Geometry check sheet. Reference: the model listing, model coordinates, mm. A direction names the side the tool comes from. Round coordinates to 2 decimals unless told otherwise and drop trailing zeros. Loops run counter-clockwise (first coordinate to the right, second up) from the corner with the lowest first, then second, coordinate; pieces in that order, holes last. Notation, with made-up numbers: (58.25, 81.5) -> (67.25, 81.5) arc R22 cw to (67.25, 94.5) -> close; hole circle Ø6 at (21, 14.25). An arc over 180 degrees is marked (long way). Use one line per item in the form item = value.
from build123d import *

# Parameters (mm, degrees)
F1_DEPTH = 25.4
F3_DEPTH = 3.176


with BuildPart() as f1:
    # F0 (on Front) → F1 (new body)
    with BuildSketch(Plane.XZ):
        with BuildLine():
            ThreePointArc((3.175, 3.175), (0.929936, 2.245064), (0, 0))
            Line((0, 0), (76.2, 0))
            Line((76.2, 0), (76.2, 76.2))
            ThreePointArc((76.2, 76.2), (73.954936, 75.270064), (73.025, 73.025))
            Line((73.025, 73.025), (73.025, 6.35))
            ThreePointArc((73.025, 6.35), (72.095064, 4.104936), (69.85, 3.175))
            Line((69.85, 3.175), (3.175, 3.175))
        make_face()
    extrude(amount=F1_DEPTH)

    # F2 (on face) → F3 (cut, through all)
    with BuildSketch(Plane.XY.offset(3.175)):
        with BuildLine():
            Line((55.5625, -9.525), (17.4625, -9.525))
            ThreePointArc((17.4625, -9.525), (14.2875, -12.7), (17.4625, -15.875))
            Line((17.4625, -15.875), (55.5625, -15.875))
            ThreePointArc((55.5625, -15.875), (58.7375, -12.7), (55.5625, -9.525))
        make_face()
    extrude(amount=-F3_DEPTH, mode=Mode.SUBTRACT)


solid = f1.part
1. Tool access check on faces 4 (the cylindrical face through (14.29, -12.63, 1.61)), 5 (the flat face through (38, -7, 0)), 6 (the flat face through (73.025, -13, 40)). Record the directions out of +Z, -Z, +X, -X, +Y, -Y that give a thin tool (end or side, any length) a straight path to the whole face; none if there is none.
Return value:
face_4 = +Z, -Z
face_5 = -Z, +X, -X, +Y, -Y
face_6 = +Z, -X, +Y, -Y
2. Material ranges on line 1 along X through (y, z) = (-13.75, 27) (3 decimals); line 2 along Z through (x, y) = (16, -18.5) (3 decimals), recorded low to high.
Return value:
line_1 = 73.025 to 76.2
line_2 = 0 to 3.175
3. Section check D-D (x = 57.5). Record the boundary of the cut face in (y, z) (3 decimals).
Return value:
outline = (-25.4, 0) -> (-15.215, 0) -> (-15.215, 3.175) -> (-25.4, 3.175) -> close; (-10.185, 0) -> (0, 0) -> (0, 3.175) -> (-10.185, 3.175) -> close
4. Mould release check, pull along Y, two halves, no side actions. Record for faces 1 (the flat face through (55, 0, 2)), 2 (the cylindrical face through (0.955, -12.522, 2.27)), 3 (the cylindrical face through (58.737, -12.77, 1.61)): released by +Y, released by -Y, zero draft, split by the parting line, or undercut.
Return value:
face_1 = released by +Y
face_2 = zero draft
face_3 = undercut
5. Section check C-C (y = -19.25). Record the boundary of the cut face in (x, z) (3 decimals).
Return value:
outline = (0, 0) -> (76.2, 0) -> (76.2, 76.2) arc R3.175 ccw to (73.025, 73.025) -> (73.025, 6.35) arc R3.175 cw to (69.85, 3.175) -> (3.175, 3.175) arc R3.175 ccw to start
6. Gauge pin test, flat ends, axial feed: pin 1 (7.5 mm diameter, centred on y = -15, z = 49, fed in from -X) (3 decimals); pin 2 (1 mm diameter, centred on x = 52, y = -6, fed in from +Z) (3 decimals). Record the tip position at first contact, or that the pin passes through.
Return value:
pin_1 = 73.025
pin_2 = 3.175
7. Section check B-B (x = 40). Record the boundary of the cut face in (y, z) (3 decimals).
Return value:
outline = (-25.4, 0) -> (-15.875, 0) -> (-15.875, 3.175) -> (-25.4, 3.175) -> close; (-9.525, 0) -> (0, 0) -> (0, 3.175) -> (-9.525, 3.175) -> close
